from build123d import *

# Parameters (mm, degrees)
F0_W                 = 110
F0_H                 = 50
F1_DEPTH             = 25
F6_D                 = 30
F7_D                 = 35
F8_D                 = 6.8
F8_DEPTH             = 28.25
F8_TIP               = 2.0429261047
F8_ON_F2_D           = 6.8
F8_ON_F2_DEPTH       = 28.25
F8_ON_F2_TIP         = 2.0429261047
F9_D                 = 8.4
F9_DEPTH             = 25
F9_CBORE_D           = 14.25
F9_CBORE_DEPTH       = 8
F9_TIP               = 2.5236145999
F9_ON_F5_D           = 8.4
F9_ON_F5_DEPTH       = 25
F9_ON_F5_CBORE_D     = 14.25
F9_ON_F5_CBORE_DEPTH = 8
F9_ON_F5_TIP         = 2.5236145999
F11_W                = 50
F11_H                = 1
F12_DEPTH            = 25
F10_W                = 1
F10_H                = 50
F13_DEPTH            = 25.0000003725
F14_D                = 6.8
F14_DEPTH            = 28.75
F14_TIP              = 2.0429261047
F14_ON_F3_D          = 6.8
F14_ON_F3_DEPTH      = 28.75
F14_ON_F3_TIP        = 2.0429261047


with BuildPart() as f1:
    # F0 (on Top) → F1 (new body, symmetric)
    with BuildSketch(Plane.XY):
        Rectangle(F0_W, F0_H)
    extrude(amount=F1_DEPTH, both=True)

    # F6 (through all)
    with Locations(Plane.XZ.offset(25)):
        with Locations((-26, 0)):
            Hole(F6_D / 2)

    # F7 (through all)
    with Locations(Plane.XY.offset(25)):
        with Locations((23, 0)):
            Hole(F7_D / 2)

    # F8
    with Locations(Plane(origin=(0, 0, -25), x_dir=(1, 0, 0), z_dir=(0, 0, -1))):
        with Locations((-47, -17), (-47, 17)):
            Hole(F8_D / 2, depth=F8_DEPTH)
            with Locations((0, 0, -(F8_DEPTH + F8_TIP / 2))):  # 118° drill point
                Cone(0, F8_D / 2, F8_TIP, mode=Mode.SUBTRACT)

    # F8 on F2
    with Locations(Plane.XZ.offset(25)):
        with Locations((47, 17), (47, -17)):
            Hole(F8_ON_F2_D / 2, depth=F8_ON_F2_DEPTH)
            with Locations((0, 0, -(F8_ON_F2_DEPTH + F8_ON_F2_TIP / 2))):  # 118° drill point
                Cone(0, F8_ON_F2_D / 2, F8_ON_F2_TIP, mode=Mode.SUBTRACT)

    # F9
    with Locations(Plane.XY.offset(25)):
        with Locations((-47, 17), (-47, -17)):
            CounterBoreHole(F9_D / 2, F9_CBORE_D / 2, F9_CBORE_DEPTH, depth=F9_DEPTH)
            with Locations((0, 0, -(F9_DEPTH + F9_TIP / 2))):  # 118° drill point
                Cone(0, F9_D / 2, F9_TIP, mode=Mode.SUBTRACT)

    # F9 on F5
    with Locations(Plane(origin=(0, 25, 0), x_dir=(-1, 0, 0), z_dir=(0, 1, 0))):
        with Locations((-47, 17), (-47, -17)):
            CounterBoreHole(F9_ON_F5_D / 2, F9_ON_F5_CBORE_D / 2, F9_ON_F5_CBORE_DEPTH, depth=F9_ON_F5_DEPTH)
            with Locations((0, 0, -(F9_ON_F5_DEPTH + F9_ON_F5_TIP / 2))):  # 118° drill point
                Cone(0, F9_ON_F5_D / 2, F9_ON_F5_TIP, mode=Mode.SUBTRACT)

    # F11 (on face) → F12 (cut)
    with BuildSketch(Plane(origin=(-55, 0, 0), x_dir=(0, -1, 0), z_dir=(-1, 0, 0))):
        Rectangle(F11_W, F11_H)
    extrude(amount=-F12_DEPTH, mode=Mode.SUBTRACT)

    # F10 (on face) → F13 (cut)
    with BuildSketch(Plane.YZ.offset(55)):
        Rectangle(F10_W, F10_H)
    extrude(amount=-F13_DEPTH, mode=Mode.SUBTRACT)

    # F14
    with Locations(Plane(origin=(0, 25, 0), x_dir=(-1, 0, 0), z_dir=(0, 1, 0))):
        with Locations((-47, 0)):
            Hole(F14_D / 2, depth=F14_DEPTH)
            with Locations((0, 0, -(F14_DEPTH + F14_TIP / 2))):  # 118° drill point
                Cone(0, F14_D / 2, F14_TIP, mode=Mode.SUBTRACT)

    # F14 on F3
    with Locations(Plane.XY.offset(25)):
        with Locations((-47, 0)):
            Hole(F14_ON_F3_D / 2, depth=F14_ON_F3_DEPTH)
            with Locations((0, 0, -(F14_ON_F3_DEPTH + F14_ON_F3_TIP / 2))):  # 118° drill point
                Cone(0, F14_ON_F3_D / 2, F14_ON_F3_TIP, mode=Mode.SUBTRACT)


solid = f1.part
Design review of the part built by this model. Coordinates are the model's own, in mm. A direction names the side the tool comes from. Give positions to 0.01 mm unless a question says otherwise; leave off trailing zeros. Loops run counter-clockwise (first coordinate to the right, second up) from the corner with the lowest first, then second, coordinate; pieces in that order, holes last. Notation, with made-up numbers: M -38.75,51 L -13.75,51 A20 cw -13.75,76 Z; hole C 60,-33.75 d11. An arc over 180 degrees is marked long. Answer as a JSON object with one key per item and string values.
Item 1: We need section C-C (x = 34). State the section outline as (y, z) points, and give its area (3 significant figures).
Output values:
{"outline": "M -25,-25 L -13.61,-25 L -13.61,25 L -25,25 Z; M 13.61,-25 L 25,-25 L 25,25 L 13.61,25 Z", "area": "1,140 mm2"}
Item 2: Wall thickness on line 1 along Z through (x, y) = (47, 6); line 2 along Y through (x, z) = (-47, 19) (3 decimals); line 3 along Y through (x, z) = (-47, -8): over which ranges is each line inside the solid? List them lowest first.
Output values:
{"line 1": "z = -25 to -21.2, -12.8 to -3.4, 3.4 to 12.8, 21.2 to 25", "line 2": "y = -25 to -24.125, -9.875 to -3.4, 3.4 to 9.875, 24.125 to 25", "line 3": "y = -25 to -20.4, -13.6 to 13.6, 20.4 to 25"}
Item 3: Mouldability with a two-part tool opening along Z and no side actions: class faces 1 (the face through (-1, 25, 0)), 2 (the face through (43.9, 17, 13.9)), 3 (the face through (-1, 0, 25)) as pulls with the +Z half, pulls with the -Z half, needs draft (parallel to the pull), parting line crosses it, or undercut.
Output values:
{"face 1": "needs draft", "face 2": "undercut", "face 3": "pulls with the +Z half"}
Item 4: We need section A-A (x = 23). State the section outline as (y, z) points, and give its area (3 significant figures).
Output values:
{"outline": "M -25,-25 L -17.5,-25 L -17.5,25 L -25,25 Z; M 17.5,-25 L 25,-25 L 25,25 L 17.5,25 Z", "area": "750 mm2"}
Item 5: Machinability: for faces 4 (the face through (-43.9, 13.9, 17)), 5 (the face through (43.9, 17, -20.1)), 6 (the face through (-55, 0, 13)), which of the approach directions +Z, -Z, +X, -X, +Y, -Y give a long, thin tool a straight path to every point of the face, cutting with its end or side? Answer none if there is none.
Output values:
{"face 4": "+Z", "face 5": "+Y", "face 6": "+Z, -Z, -X, +Y, -Y"}
Item 6: For P1, Ø9, axis at x = -47, y = 17, coming from the -Z side; P2, Ø11, axis at x = -47, y = -17, coming from the +Z side; P3, Ø4.5, axis at x = 46, z = 15, coming from the +Y side; P4, Ø8, axis at x = -28.5, z = -8.5, coming from the -Y side, all flat-tipped, find the tip position at first contact; note any pin that passes through.
Output values:
{"P1": "stops at z = -25", "P2": "stops at z = 17", "P3": "stops at y = 17", "P4": "passes through"}
Item 7: We need section B-B (z = 19). State the section outline as (x, y) points (3 decimals).
Output values:
{"outline": "M -55,-25 L 44.25,-25 L 44.25,-0.5 L 40.493,-0.5 A17.5 cw long 40.493,0.5 L 43.307,0.5 L 43.307,17 L 40.161,17 L 40.161,25 L -55,25 Z; M 49.75,-25 L 55,-25 L 55,-0.5 L 49.75,-0.5 Z; M 50.693,0.5 L 55,0.5 L 55,25 L 53.839,25 L 53.839,17 L 50.693,17 Z; hole C -47,-17 d14.25; hole C -47,17 d14.25; hole C -47,0 d6.8"}
